Read the model definition and answer for the solid it produces. Units are mm, in the model's axes. Give positions to 0.01 mm unless a question says otherwise; leave off trailing zeros. Order: outer loops, then holes, each group sorted by start corner. A loop starts at its lowest first (then second) coordinate and runs counter-clockwise, first axis right, second up. Notation, with made-up numbers: (-19, 86.5) -> (9, 86.5) arc R19 ccw to (9, 107.5) -> close; hole circle Ø1 at (40.25, 34.25). An arc over 180 degrees is marked (long way). One line per question, with ' | ' between items. Start each with the question number.
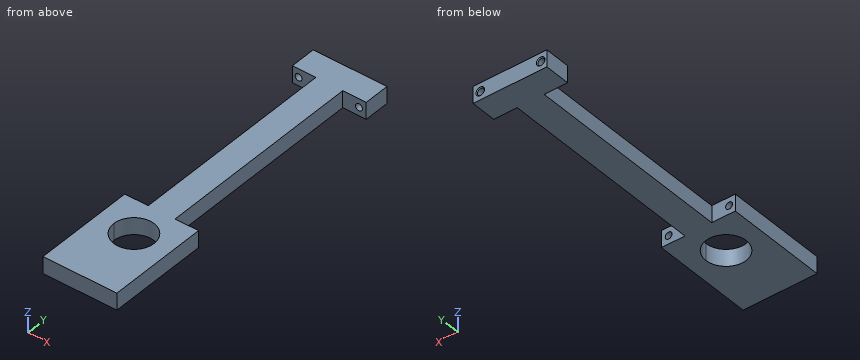
```python
from build123d import *
from build123d.topology import SkipClean

# Parameters (mm, degrees)
EXTRUDE_1_DEPTH                = 5
EXTRUDE_2_DEPTH                = 5
EXTRUDE_START                  = -5
EXTRUDE_3_DEPTH                = 5
HOLE_WIZARD_M2_5_1_D           = 2.05
HOLE_WIZARD_M2_5_1_CSINK_D     = 2.55
HOLE_WIZARD_M2_5_1_CSINK_ANGLE = 90
SKETCH_7_W                     = 22
SKETCH_7_H                     = 10
EXTRUDE_4_DEPTH                = 5


with BuildPart() as part:
    # 草图1 → 凸台-拉伸1 (new body)
    with BuildSketch(Plane.XY):
        with BuildLine():
            Line((-6, 0), (-11, 0))
            Line((-11, 0), (-11, 10.250706887))
            Line((-11, 10.250706887), (11, 10.250706887))
            Line((11, 10.250706887), (11, 0))
            Line((11, 0), (6, 0))
            ThreePointArc((6, 0), (0, 6), (-6, 0))
        make_face()
    extrude(amount=EXTRUDE_1_DEPTH)

    # 草图2 → 凸台-拉伸2 (add)
    with BuildSketch(Plane.XY.offset(5)):
        Polygon((4, 72.311119812), (4, 10.250706887), (-4, 10.250706887), (-4, 72.311119812), (-11, 72.311119812), (-11, 80), (11, 80), (11, 72.311119812), align=None)
    extrude(amount=-EXTRUDE_2_DEPTH)

    # 草图6 → 凸台-拉伸3 (add)
    with SkipClean():  # the faces are left unmerged after this step: merging them gives an invalid solid
        with BuildSketch(Plane(origin=(0, 0, 0), x_dir=(-1, 0, 0), z_dir=(0, 0, -1)).offset(EXTRUDE_START)):
            with BuildLine():
                Line((-11, 0), (-11, -10))
                Line((-11, -10), (11, -10))
                Line((11, -10), (11, 0))
                Line((11, 0), (6, 0))
                ThreePointArc((6, 0), (0, -6), (-6, 0))
                Line((-6, 0), (-11, 0))
            make_face()
        extrude(amount=EXTRUDE_3_DEPTH)
    add(part.part.scale(1), mode=Mode.REPLACE)  # the faces are merged on a copy

    # M2.5 螺纹孔1 (through all)
    with Locations(Plane(origin=(0, 80, 0), x_dir=(1, 0, 0), z_dir=(0, 1, 0))):
        with Locations((-9.154712184, -2.5), (8.845287816, -2.5)):
            CounterSinkHole(HOLE_WIZARD_M2_5_1_D / 2, HOLE_WIZARD_M2_5_1_CSINK_D / 2, counter_sink_angle=HOLE_WIZARD_M2_5_1_CSINK_ANGLE)

    # 草图7 → 凸台-拉伸4 (add)
    with BuildSketch(Plane.XY.offset(5)):
        with Locations((0, -15)):
            Rectangle(SKETCH_7_W, SKETCH_7_H)
    extrude(amount=-EXTRUDE_4_DEPTH)


solid = part.part
```
Q1. A cutting plane is placed at A-A, the plane z = 2.5. Give the number of separate pieces and of enclosed holes in the cut face, then the cut area to 3 significant figures.
Q2. Given P1, Ø0.6, axis at x = 8.5, z = 2.5, coming from the +Y side; P2, Ø2, axis at y = 22.5, z = 3.5, coming from the -X side, each flat-ended and moving along its own axis, determine where each tip first touches the part or whether it passes through.
Q3. A cutting plane is placed at C-C, the plane y = -7. Determine the outline of the cut face in (x, z) (3 decimals).
Q4. A cutting plane is placed at D-D, the plane y = 54. Determine the outline of the cut face in (x, z).
Q5. Find the intervals of material crossed by line 1 (Y direction, x = -8.75, z = 4.75); line 2 (Y direction, x = -4.5, z = 3.8); line 3 (X direction, y = 11.5, z = 3.3), in increasing order.
Q6. A cutting plane is placed at B-B, the plane x = 0. Determine the outline of the cut face in (y, z), then the cut area to 3 significant figures.
Geometry results:
1) separate pieces: 3 | enclosed holes: 1 | area: 1,100 mm²
2) P1: y = -10 | P2: x = -4
3) outline: (-11, 0) -> (11, 0) -> (11, 5) -> (-11, 5) -> close; hole circle Ø2.05 at (-9.155, 2.5); hole circle Ø2.05 at (8.845, 2.5)
4) outline: (-4, 0) -> (4, 0) -> (4, 5) -> (-4, 5) -> close
5) line 1: -20 to 10.25, 72.31 to 80 | line 2: -20 to -3.97, 3.97 to 10.25, 72.31 to 80 | line 3: -4 to 4
6) outline: (-20, 0) -> (-6, 0) -> (-6, 5) -> (-20, 5) -> close; (6, 0) -> (80, 0) -> (80, 5) -> (6, 5) -> close | area: 440 mm²
